The model under review builds one solid part; all positions refer to its coordinate system, in mm. A direction names the side the tool comes from. Round coordinates to 2 decimals unless told otherwise and drop trailing zeros. Write each loop counter-clockwise with the first axis right and the second up, starting at its lowest first coordinate (ties: lowest second). Pieces come first, ordered by that corner, then holes. Notation, with made-up numbers: (9.5, 36) - (67.5, 36) arc R32 cw to (67.5, 62) - close; hole circle Ø8 at (85.5, 67.5). An arc over 180 degrees is marked (long way). Write each question's results on one line, items separated by ' | '.
```python
from build123d import *

# Parameters (mm, degrees)
SKETCH1_R                     = 12.9
BOSS_EXTRUDE1_DEPTH           = 2
SKETCH2_R                     = 12.9
BOSS_EXTRUDE2_DEPTH           = 4.5
BOSS_EXTRUDE2_TAPER           = 45
SKETCH3_R                     = 8.4
BOSS_EXTRUDE3_DEPTH           = 23.5
SKETCH5_R                     = 8.4
BOSS_EXTRUDE4_DEPTH           = 3
BOSS_EXTRUDE4_TAPER           = 21.8
F_6_0MM_START                 = -6.501
F_6_0MM_DOWEL_HOLE1_OUTLINE_R = 1.5
F_6_0MM_DOWEL_HOLE1_DEPTH     = 6.501


# Read off the part's stored shape, not the designer's step: Ø6.0mm Dowel Hole1
with BuildPart() as part:
    # Sketch1 → Boss-Extrude1 (new body)
    with BuildSketch(Plane(origin=(0, 0, 0), x_dir=(1, 0, 0), z_dir=(0, 1, 0))):
        with Locations(Location((0, 0, 0), (0, 0, 270))):
            Circle(SKETCH1_R)
    extrude(amount=-BOSS_EXTRUDE1_DEPTH)

    # Sketch2 → Boss-Extrude2 (add)
    with BuildSketch(Plane.XZ.offset(2)):
        with Locations(Location((0, 0, 0), (0, 0, 90))):
            Circle(SKETCH2_R)
    extrude(amount=BOSS_EXTRUDE2_DEPTH, taper=BOSS_EXTRUDE2_TAPER)

    # Sketch3 → Boss-Extrude3 (add)
    with BuildSketch(Plane.XZ.offset(6.5)):
        with Locations(Location((0, 0, 0), (0, 0, 270))):
            Circle(SKETCH3_R)
    extrude(amount=BOSS_EXTRUDE3_DEPTH)

    # Sketch5 → Boss-Extrude4 (add)
    with BuildSketch(Plane.XZ.offset(30)):
        with Locations(Location((0, 0, 0), (0, 0, 270))):
            Circle(SKETCH5_R)
    extrude(amount=BOSS_EXTRUDE4_DEPTH, taper=BOSS_EXTRUDE4_TAPER)

    # Ø6.0mm Dowel Hole1 outline → Ø6.0mm Dowel Hole1 (cut)
    with BuildSketch(Plane(origin=(0, 0, 0), x_dir=(1, 0, 0), z_dir=(0, 1, 0)).offset(F_6_0MM_START)):
        with Locations((4.5, -7.794228634)):
            Circle(F_6_0MM_DOWEL_HOLE1_OUTLINE_R)
        with Locations((4.5, 7.794228634)):
            Circle(F_6_0MM_DOWEL_HOLE1_OUTLINE_R)
        with Locations((-9, 0)):
            Circle(F_6_0MM_DOWEL_HOLE1_OUTLINE_R)
    extrude(amount=F_6_0MM_DOWEL_HOLE1_DEPTH, mode=Mode.SUBTRACT)


solid = part.part
```
Q1. We need section C-C (x = 4.5). State how many separate pieces and enclosed holes the cut face has, plus the area to 3 significant figures.
Evaluation:
separate pieces: 3 | enclosed holes: 0 | area: 472 mm^2
Q2. Insertion check: P1, Ø4, axis at y = -17, z = -2, coming from the +X side; P2, Ø3, axis at x = -1.5, y = -29, coming from the +Z side; P3, Ø1, axis at x = 5, y = -4, coming from the -Z side. Each pin has a flat end and moves straight along its axis. Give the tip position at first contact, or say it passes through.
Evaluation:
P1: stops at x = 8.4 | P2: stops at z = 8.4 | P3: stops at z = -10.29
Q3. We need section A-A (z = 0). State the section outline as (x, y) points.
Evaluation:
outline: (-12.9, -2) - (-10.5, -4.4) - (-10.5, 0) - (-12.9, 0) - close; (-8.4, -30) - (-7.2, -33) - (7.2, -33) - (8.4, -30) - (8.4, -6.5) - (12.9, -2) - (12.9, 0) - (-7.5, 0) - (-7.5, -6.5) - (-8.4, -6.5) - close
Q4. We need section B-B (y = -28). State the section outline as (x, z) points.
Evaluation:
outline: circle Ø16.8 at (0, 0)
Q5. For probe 1 along Z at (x, y) = (4.5, -3.5); probe 2 along Z at (x, y) = (4.5, -1.25); probe 3 along Z at (x, y) = (3, -26), list the stretches that pass through material, from the lowest coordinate up.
Evaluation:
probe 1: z = -10.47 to -9.29, -6.29 to 6.29, 9.29 to 10.47 | probe 2: z = -12.09 to -9.29, -6.29 to 6.29, 9.29 to 12.09 | probe 3: z = -7.85 to 7.85
Q6. Tool access review of faces 1 (the cylindrical face through (-12.593, -0.986, -2.796)), 2 (the flat face through (-8, -6.501, 0)), 3 (the cylindrical face through (3.394, -2.574, 6.78)): name each direction out of +Z, -Z, +X, -X, +Y, -Y from which nothing blocks a thin tool from reaching the whole face with its end or side.
Evaluation:
face 1: +Y, -Y | face 2: -X, +Y | face 3: +Y
Q7. The part is to be moulded in two halves that separate along Z. For faces 4 (the cylindrical face through (4.17, -2.57, -6.33)), 5 (the cylindrical face through (2.523, -18.086, -8.012)), 6 (the flat face through (4, -6.501, 7)), 7 (the cylindrical face through (-7.57, -2.57, -0.45)), say which applies: released by +Z, released by -Z, zero draft, split by the parting line, or undercut.
Evaluation:
face 4: undercut | face 5: split by the parting line | face 6: zero draft | face 7: undercut
